Work out the finished part from the listing and answer in its coordinate system (mm). Face numbers are marked on the shaded views. A direction names the side the tool comes from. Coordinates: 2 decimals unless noted, no trailing zeros. Order: outer loops, then holes, each group sorted by start corner. A loop starts at its lowest first (then second) coordinate and runs counter-clockwise, first axis right, second up. Notation, with made-up numbers: M -31,-3 L -27,-3 A19 ccw -27,2 Z; hole C 6,43 d9. An arc over 180 degrees is marked long. Write item = value, one per line. Start each with the question number.
Q1. Find section C-C on z = -21. Give the vertices of the cut face in (x, y), and give its area (3 significant figures).
Q2. Straight lines are drawn through the part: line 1 along Y through (x, z) = (0, -15.55); line 2 along X through (y, z) = (4.5, -15.5); line 3 along Z through (x, y) = (8.5, 12). For each, find the intervals that lie inside material, in ascending order.
Q3. Each of these flat-tipped pins is pushed along its axis until it touches: P1, Ø0.8, axis at x = -3, y = -0.5, coming from the +Z side; P2, Ø2, axis at x = 10.61, y = -10.61, coming from the +Z side; P3, Ø3, axis at y = -2, z = -36, coming from the +X side. Where does it stop, or does it pass through?
Q4. Find section B-B on z = -36. Give the vertices of the cut face in (x, y).
Q5. A tool of negligible diameter and unlimited length cuts with its end or side. For the marked faces 1, 2 and 3, from which of +Z, -Z, +X, -X, +Y, -Y can it reach the whole face along a straight path? Write none if from no direction.
Q6. Find section D-D on z = -7.5. Give the vertices of the cut face in (x, y), and give its area (3 significant figures).
```python
from build123d import *

# Parameters (mm, degrees)
FILLET3_R                      = 2
CUT_EXTRUDE11_START            = -10
CUT_EXTRUDE11_DEPTH            = 10
CHAMFER6_SIZE                  = 0.5
M3X0_5_TAPPED_HOLE1_AT_2_COUNT = 2
M3X0_5_TAPPED_HOLE1_AT_2_PITCH = 11.136209045
CIRPATTERN4_COUNT              = 3
SKETCH43_R                     = 1.25
EXTRUDE13_DEPTH                = 15
CUT_EXTRUDE13_START            = -5
SKETCH44_R                     = 20
SKETCH44_R_2                   = 19.99
CUT_EXTRUDE13_DEPTH            = 5


with BuildPart() as part:
    # Sketch37 → Revolve3 (revolve)
    with BuildSketch(Plane(origin=(0, 0, 0), x_dir=(0, 0, -1), z_dir=(1, 0, 0)), mode=Mode.PRIVATE) as revolve3_sk:
        Polygon((0, 0), (0, -4), (14.9, -4), (14.9, -5), (15.9, -5), (15.9, -7.5), (14.9, -7.5), (14.9, -10), (19.9, -10), (19.9, -20), (51, -20), (51, 0), align=None)
    revolve(revolve3_sk.sketch.rotate(Axis((0, 0, 0), (0, 0, -1)), 270), axis=Axis((0, 0, 0), (0, 0, -1)))

    # Fillet3
    fillet3_edges = [part.edges().sort_by_distance(p)[0] for p in [
        (-20, 0, -51),
    ]]
    fillet(fillet3_edges, radius=FILLET3_R)

    # Sketch38 → Cut-Extrude11 (cut)
    with BuildSketch(Plane.XY.offset(CUT_EXTRUDE11_START)):
        with BuildLine():
            Line((-2.5, 3.122498999), (-2.5, -3.122498999))
            ThreePointArc((-2.5, -3.122498999), (-4, 0), (-2.5, 3.122498999))
        make_face()
    extrude(amount=CUT_EXTRUDE11_DEPTH, mode=Mode.SUBTRACT)

    # Chamfer6
    chamfer6_edges = [part.edges().sort_by_distance(p)[0] for p in [
        (-10, 0, -14.9),
        (-7.5, 0, -14.9),
        (1.732050808, 3.605551275, 0),
        (-20, 0, -19.9),
    ]]
    chamfer(chamfer6_edges, length=CHAMFER6_SIZE)

    # Sketch40 → M3x0.5 Tapped Hole1 (revolve, cut)
    with BuildSketch(Plane(origin=(0, -14, -19.9), x_dir=(0, -1, 0), z_dir=(1, 0, 0))):
        Polygon((0, 0), (0, 9.251075774), (1.25, 8.5), (1.25, 0), align=None)
    m3x0_5_tapped_hole1 = revolve(axis=Axis((0, -14, -13.55), (0, 0, -1)), mode=Mode.SUBTRACT)

    # M3x0.5 Tapped Hole1 at 2: M3x0.5 Tapped Hole1 ×2
    with Locations(*[Vector(0.9524427634762035, 0.30471754511647786, 0) * (i * M3X0_5_TAPPED_HOLE1_AT_2_PITCH) for i in range(1, M3X0_5_TAPPED_HOLE1_AT_2_COUNT)]):
        add(m3x0_5_tapped_hole1, mode=Mode.SUBTRACT)

    # CirPattern4: M3x0.5 Tapped Hole1 ×3 about axis
    cirpattern4_axis = Axis((0, 0, 0), (0, 0, 1))
    for i in range(1, CIRPATTERN4_COUNT):
        add(m3x0_5_tapped_hole1.rotate(cirpattern4_axis, i * 360 / CIRPATTERN4_COUNT), mode=Mode.SUBTRACT)

    # CirPattern4 copy 1 sketch → CirPattern4 copy 1 (revolve, cut)
    with BuildSketch(Plane(origin=(3.882285677, 14.488887394, -19.9), x_dir=(0.8660254037844387, 0.4999999999999998, 0), z_dir=(-0.4999999999999998, 0.8660254037844387, 0))):
        Polygon((0, 0), (0, 9.251075774), (1.25, 8.5), (1.25, 0), align=None)
    revolve(axis=Axis((3.882285677, 14.488887394, -13.55), (0, 0, -1)), mode=Mode.SUBTRACT)

    # CirPattern4 copy 2 sketch → CirPattern4 copy 2 (revolve, cut)
    with BuildSketch(Plane(origin=(-14.488887394, -3.882285677, -19.9), x_dir=(-0.8660254037844384, 0.5000000000000004, 0), z_dir=(-0.5000000000000004, -0.8660254037844384, 0))):
        Polygon((0, 0), (0, 9.251075774), (1.25, 8.5), (1.25, 0), align=None)
    revolve(axis=Axis((-14.488887394, -3.882285677, -13.55), (0, 0, -1)), mode=Mode.SUBTRACT)

    # Sketch43 → Extrude13 (add)
    with BuildSketch(Plane.XY.offset(-19.9)):
        with Locations((0, -14)):
            Circle(SKETCH43_R)
        with Locations((-12.124355653, 7)):
            Circle(SKETCH43_R)
        with Locations((12.124355653, 7)):
            Circle(SKETCH43_R)
    extrude(amount=-EXTRUDE13_DEPTH)

    # Sketch44 → Cut-Extrude13 (cut)
    with BuildSketch(Plane.XY.offset(-19.9).offset(CUT_EXTRUDE13_START)):
        Circle(SKETCH44_R)
        Circle(SKETCH44_R_2, mode=Mode.SUBTRACT)
    extrude(amount=CUT_EXTRUDE13_DEPTH, mode=Mode.SUBTRACT)


solid = part.part
```
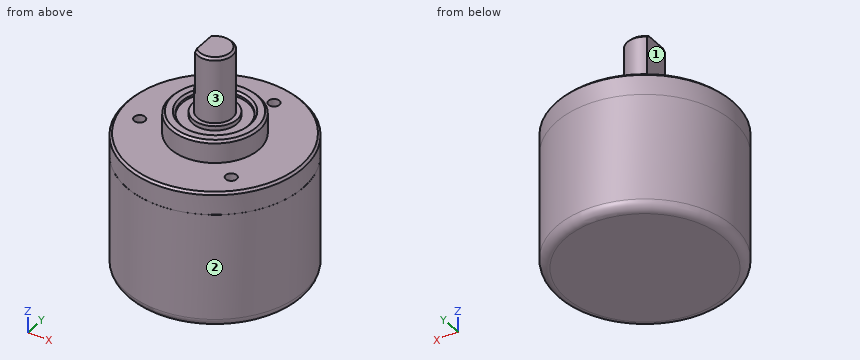
Findings below:
q1.outline = C 0,0 d39.98; hole C -14.49,-3.88 d2.5; hole C 3.88,14.49 d2.5; hole C 10.61,-10.61 d2.5
q1.area = 1,240 mm^2
q2.line_1 = -10 to -7.5, -5 to 5, 7.5 to 10
q2.line_2 = -8.93 to -6, -2.18 to 2.18, 6 to 8.93
q2.line_3 = -51 to -19.9
q3.P1 = -10
q3.P2 = -28.55
q3.P3 = 19.99
q4.outline = C 0,0 d40
q5.face_1 = +Z, -X, +Y, -Y
q5.face_2 = +Z, -Z
q5.face_3 = +Z
q6.outline = M -2.5,-3.12 A4 ccw long -2.5,3.12 Z
q6.area = 43.7 mm^2
